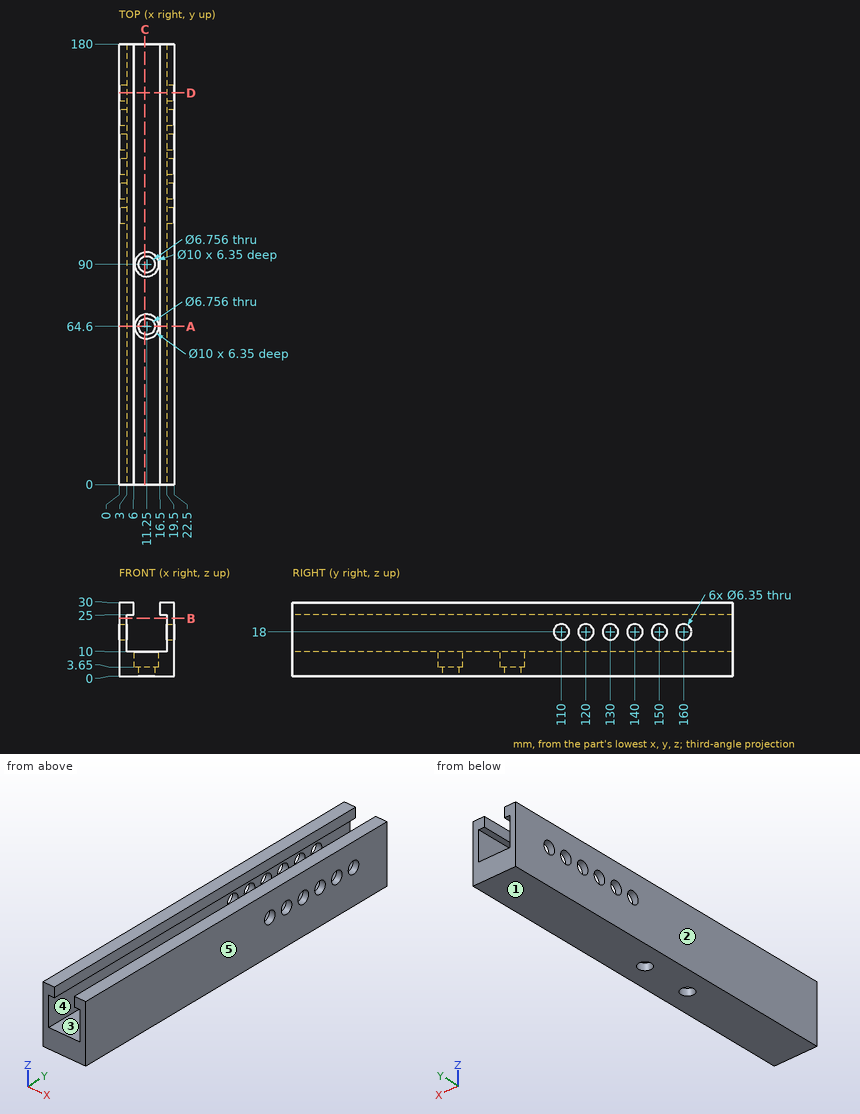
Job drawing, mm, ordinate dimensions from the low corner. One solid piece. A direction names the side the tool comes from. Give positions to 0.01 mm unless a question says otherwise; leave off trailing zeros. Order: outer loops, then holes, each group sorted by start corner. A loop starts at its lowest first (then second) coordinate and runs counter-clockwise, first axis right, second up. Notation, with made-up numbers: M 5,11.5 L 63,11.5 A28 ccw 63,46.5 Z; hole C 76,28.25 d11. An arc over 180 degrees is marked long. Put each result on its own line as item: value. Start each with the question number.
(1) Pull direction Z, two halves, no side cores. Call the marked faces 1, 2 and 3: released by +Z, released by -Z, zero draft, split by the parting line, or undercut.
(2) Band-saw the part on C-C on x = 10.5. Give the cut face in (y, z).
(3) Drill centre lines: L1, parallel to Y at x = 11.25, z = 2.5; L2, parallel to X at y = 144, z = 14; L3, parallel to Z at x = 21.05, y = 160 (1 decimal). Where is each one in solid material? Low to high. Write a range as [from, to].
(4) Band-saw the part on D-D on y = 160. Give the cut face in (x, z) (1 decimal), then the cut area to 3 significant figures.
(5) Band-saw the part on B-B on z = 23.5. Give the cut face in (x, y), then the cut area to 3 significant figures.
(6) Band-saw the part on A-A on y = 64.6. Give the cut face in (x, z).
(7) Pin check, flat tip, straight feed: pin 1 Ø9 at (x, y) = (11.25, 64.6) entering from +Z. Stop position of the tip, or through.
(8) Tool access for the marked faces 4 and 5: list every direction of +Z, -Z, +X, -X, +Y, -Y with a clear straight run to the whole face (end or side of a thin tool).
Results below:
1. face 1: released by -Z
1. face 2: zero draft
1. face 3: undercut
2. outline: M 0,0 L 61.31,0 L 61.31,3.65 L 59.66,3.65 L 59.66,10 L 0,10 Z; M 67.89,0 L 86.71,0 L 86.71,3.65 L 85.06,3.65 L 85.06,10 L 69.54,10 L 69.54,3.65 L 67.89,3.65 Z; M 93.29,0 L 180,0 L 180,10 L 94.94,10 L 94.94,3.65 L 93.29,3.65 Z
3. L1: y = [0, 61.22], [67.98, 86.62], [93.38, 180]
3. L2: x = [0, 3], [19.5, 22.5]
3. L3: z = [0, 14.8], [21.2, 30]
4. outline: M 0,0 L 22.5,0 L 22.5,14.8 L 19.5,14.8 L 19.5,10 L 3,10 L 3,14.8 L 0,14.8 Z; M 0,21.2 L 3,21.2 L 3,25 L 6,25 L 6,30 L 0,30 Z; M 16.5,25 L 19.5,25 L 19.5,21.2 L 22.5,21.2 L 22.5,30 L 16.5,30 Z
4. area: 337 mm2
5. outline: M 0,0 L 3,0 L 3,180 L 0,180 Z; M 19.5,0 L 22.5,0 L 22.5,180 L 19.5,180 Z
5. area: 1,080 mm2
6. outline: M 0,0 L 7.87,0 L 7.87,3.65 L 6.25,3.65 L 6.25,10 L 3,10 L 3,25 L 6,25 L 6,30 L 0,30 Z; M 14.63,0 L 22.5,0 L 22.5,30 L 16.5,30 L 16.5,25 L 19.5,25 L 19.5,10 L 16.25,10 L 16.25,3.65 L 14.63,3.65 Z
7. pin 1: stops at z = 3.65
8. face 4: +Y, -Y
8. face 5: +Z, -Z, +X, +Y, -Y
